CAD build for the part. Positions are in the model's coordinates, mm. Face numbers are marked on the shaded views. A direction names the side the tool comes from. Give positions to 0.01 mm unless a question says otherwise; leave off trailing zeros. Write each loop counter-clockwise with the first axis right and the second up, starting at its lowest first coordinate (ties: lowest second). Pieces come first, ordered by that corner, then holes. Notation, with made-up numbers: (-0.75, 75.25) - (8.25, 75.25) arc R16 cw to (8.25, 99.25) - close; hole circle Ø4 at (-18, 47.5). An arc over 180 degrees is marked (long way). Answer as a JSON object with one key per item and string values.
from build123d import *

# Parameters (mm, degrees)
F0_R     = 20
F1_DEPTH = 2
F4_SIZE  = 0.49999
F5_SIZE  = 1.49999


# Not quite as in the source:
# - a fillet or chamfer is up to 0.001 mm smaller than in the source, because OpenCascade refuses the exact size


with BuildPart() as f1:
    # F0 (on Top) → F1 (new body)
    with BuildSketch(Plane.XY):
        Circle(F0_R)
        with BuildLine():
            Line((-1.5, -13), (1.5, -13))
            ThreePointArc((1.5, -13), (4, -15.5), (1.5, -18))
            Line((1.5, -18), (-1.5, -18))
            ThreePointArc((-1.5, -18), (-4, -15.5), (-1.5, -13))
        make_face(mode=Mode.SUBTRACT)
        with BuildLine():
            ThreePointArc((2.5, 13.5), (0, 11), (-2.5, 13.5))
            Line((-2.5, 13.5), (-2.5, 15.5))
            ThreePointArc((-2.5, 15.5), (0, 18), (2.5, 15.5))
            Line((2.5, 15.5), (2.5, 13.5))
        make_face(mode=Mode.SUBTRACT)
    extrude(amount=F1_DEPTH)

    # F2 (on Front) → F3 (revolve)
    with BuildSketch(Plane.XZ):
        Polygon((0, 30), (0, 2), (10, 2), (10, 10), (9.5, 10), (9.5, 20), (8, 20), (9, 28), (9.5, 28), (9.5, 30), align=None)
    revolve(axis=Axis((0, 0, 44.0067852139), (0, 0, 1)))

    # F4 (size 0.5 in the source; OpenCascade refuses exactly that, so slightly less here)
    f4_edges = [f1.edges().sort_by_distance(p)[0] for p in [
        (-9.5, 0, 28),
    ]]
    chamfer(f4_edges, length=F4_SIZE)

    # F5 (size 1.5 in the source; OpenCascade refuses exactly that, so slightly less here)
    f5_edges = [f1.edges().sort_by_distance(p)[0] for p in [
        (-9.5, 0, 20),
    ]]
    chamfer(f5_edges, length=F5_SIZE)


solid = f1.part
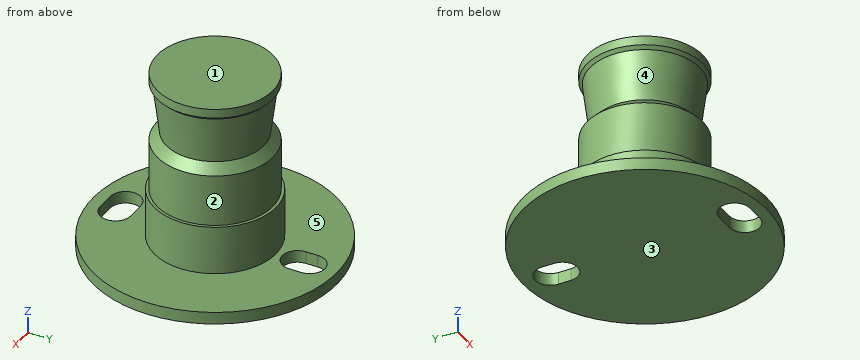
(1) Saw through at A-A, the plane x = 0. State how many separate pieces and enclosed holes the cut face has, and give its area (4 significant figures).
Answer key:
{"separate pieces": "3", "enclosed holes": "0", "area": "577.5 mm²"}
(2) Saw through at C-C, the plane z = 8. Give the cut face in (x, y).
Answer key:
{"outline": "circle Ø20 at (0, 0)"}
(3) Flat gauge pins, fed straight in: P1, Ø2, axis at y = 14, z = 1.5, coming from the -X side; P2, Ø12, axis at y = 1.5, z = 26.5, coming from the -X side; P3, Ø2, axis at x = 0.5, z = 1.5, coming from the +Y side. Where does each tip first touch, or does it go through?
Answer key:
{"P1": "stops at x = -15.2", "P2": "stops at x = -9.5", "P3": "stops at y = 20"}
(4) Pull direction Z, two halves, no side cores. Call the marked faces 3, 4 and 5: pulls with the +Z half, pulls with the -Z half, needs draft (parallel to the pull), parting line crosses it, or undercut.
Answer key:
{"face 3": "pulls with the -Z half", "face 4": "undercut", "face 5": "pulls with the +Z half"}
(5) Probe L1, parallel to Z at x = -17, y = 2; L2, parallel to Y at x = -3, z = 11.5; L3, parallel to Z at x = -9, y = -1. List the from-to ranges inside material, lowest first. Write a range as [from, to].
Answer key:
{"L1": "z = [0, 2]", "L2": "y = [-9.01, 9.01]", "L3": "z = [0, 18.94], [28.06, 30]"}
(6) 3-axis set-ups, long thin cutter, end or side, ignore diameter. For the marked faces 1 and 2: which of +Z, -Z, +X, -X, +Y, -Y reach the whole face in a straight line?
Answer key:
{"face 1": "+Z, +X, -X, +Y, -Y", "face 2": "+Z"}
(7) Saw through at D-D, the plane x = -11. Give the cut face in (y, z), and give its area (3 significant figures).
Answer key:
{"outline": "(-16.7, 0) - (16.7, 0) - (16.7, 2) - (-16.7, 2) - close", "area": "66.8 mm²"}
